Work out the finished part from the listing and answer in its coordinate system (mm). A direction names the side the tool comes from. Coordinates: 2 decimals unless noted, no trailing zeros. Order: outer loops, then holes, each group sorted by start corner. A loop starts at its lowest first (then second) coordinate and runs counter-clockwise, first axis right, second up. Notation, with made-up numbers: M -24.5,46.5 L 10.5,46.5 A29 ccw 10.5,85.5 Z; hole C 26.5,-7 d2. An arc over 180 degrees is marked long. Use a Markdown table: item, result.
from build123d import *

# Parameters (mm, degrees)
Y_KSEKLIK_EKSTR_ZYON1_DEPTH = 38
RADYUS3_R                   = 8
Y_KSEKLIK_EKSTR_ZYON2_DEPTH = 10
Y_KSEKLIK_EKSTR_ZYON3_DEPTH = 24
KES_EKSTR_ZYON1_DEPTH       = 68
KES_EKSTR_ZYON3_DEPTH       = 68
KES_EKSTR_ZYON3_DEPTH_BACK  = 68
KES_EKSTR_ZYON4_DEPTH       = 68
KES_EKSTR_ZYON7_DEPTH       = 68


with BuildPart() as part:
    # Çizim1 → Yükseklik-Ekstrüzyon1 (new body)
    with BuildSketch(Plane.XY):
        with BuildLine():
            Line((-8, 0), (-24, 0))
            Line((-24, 0), (-24, -12))
            Line((-24, -12), (-19.5, -18))
            Line((-19.5, -18), (-12.5, -18))
            Line((-12.5, -18), (-10.25, -15))
            Line((-10.25, -15), (10.25, -15))
            Line((10.25, -15), (12.5, -18))
            Line((12.5, -18), (19.5, -18))
            Line((19.5, -18), (24, -12))
            Line((24, -12), (24, 0))
            Line((24, 0), (8, 0))
            ThreePointArc((8, 0), (0, -8), (-8, 0))
        make_face()
    extrude(amount=Y_KSEKLIK_EKSTR_ZYON1_DEPTH)

    # Radyus3
    # the kernel refuses this fillet: 8 mm, written as the material it adds along each edge
    with BuildSketch(Plane(origin=(10.25, -15, 0), x_dir=(-1, 0, 0), z_dir=(0, 0, 1))) as radyus3_piece_1:
        with BuildLine():
            CenterArc((3.994997998, 8), RADYUS3_R, 218.682187453, 51.317812547)
            Line((-2.25, 3), (-2.37489996, 2.9))
            ThreePointArc((-2.37489996, 2.9), (-1.253, 1.404), (-0.128, -0.096))
            Line((-0.128, -0.096), (0, -0.16))
            Line((0, -0.16), (3.994997998, -0.16))
            Line((3.994997998, -0.16), (3.994997998, 0))
        make_face()
    extrude(amount=38)
    with BuildSketch(Plane(origin=(-10.25, -15, 0), x_dir=(-0.5999999999999978, -0.8000000000000017, 0), z_dir=(0, 0, 1))) as radyus3_piece_2:
        with BuildLine():
            CenterArc((4.003001201, 7.995998399), RADYUS3_R, 216.869897646, 51.317812547)
            Line((-2.396998799, 3.195998399), (-2.524998799, 3.099998399))
            Line((-2.524998799, 3.099998399), (-0.128, -0.096))
            Line((-0.128, -0.096), (0, -0.16))
            ThreePointArc((0, -0.16), (1.875, -0.16), (3.744939976, -0.159919968))
            Line((3.744939976, -0.159919968), (3.75, 0))
        make_face()
    extrude(amount=38)

    # Çizim2 → Yükseklik-Ekstrüzyon2 (add)
    with BuildSketch(Plane.XY.offset(38)):
        with BuildLine():
            Line((22.125, -12), (24, -12))
            Line((24, -12), (24, 0))
            Line((24, 0), (-24, 0))
            Line((-24, 0), (-24, -12))
            Line((-24, -12), (-22.125, -12))
            Line((-22.125, -12), (-18.75, -16.5))
            Line((-18.75, -16.5), (-13.183205232, -16.5))
            ThreePointArc((-13.183205232, -16.5), (-10.029919219, -14.282202113), (-6.255002002, -13.5))
            Line((-6.255002002, -13.5), (6.255002002, -13.5))
            ThreePointArc((6.255002002, -13.5), (10.029919219, -14.282202113), (13.183205232, -16.5))
            Line((13.183205232, -16.5), (18.75, -16.5))
            Line((18.75, -16.5), (22.125, -12))
        make_face()
    extrude(amount=Y_KSEKLIK_EKSTR_ZYON2_DEPTH)

    # Çizim4 → Yükseklik-Ekstrüzyon3 (add, symmetric)
    with BuildSketch(Plane(origin=(0, 0, 0), x_dir=(0, 0, -1), z_dir=(1, 0, 0))):
        Polygon((-109, -10.5), (-103, -16.5), (-48, -16.5), (-48, 0), (-98, 0), (-98, 5.5), (-103, 5.5), (-109, -0.5), align=None)
    extrude(amount=Y_KSEKLIK_EKSTR_ZYON3_DEPTH, both=True)

    # Çizim5 → Kes-Ekstrüzyon1 (cut)
    with BuildSketch(Plane(origin=(0, 0, 48), x_dir=(-1, 0, 0), z_dir=(0, 0, -1))):
        Polygon((24, -16.5), (24, -12), (22.125, -12), (18.75, -16.5), align=None)
    extrude(amount=-KES_EKSTR_ZYON1_DEPTH, mode=Mode.SUBTRACT)

    # Çizim6 → Kes-Ekstrüzyon3 (cut, two sides: drawn at the far end of the back side and taken through both)
    with BuildSketch(Plane(origin=(0, 0, 0), x_dir=(1, 0, 0), z_dir=(0, 1, 0)).offset(-KES_EKSTR_ZYON3_DEPTH_BACK)):
        Polygon((-24, -83.22), (-34.13268128, -83.22), (-34.13268128, -122.200491655), (32.816911355, -122.200491655), (32.816911355, -83.22), (24, -83.22), (12, -104.004609691), (-12, -104.004609691), align=None)
    extrude(amount=KES_EKSTR_ZYON3_DEPTH + KES_EKSTR_ZYON3_DEPTH_BACK, mode=Mode.SUBTRACT)

    # Çizim7 → Kes-Ekstrüzyon4 (cut)
    with BuildSketch(Plane(origin=(0, 0, 48), x_dir=(-1, 0, 0), z_dir=(0, 0, -1))):
        with BuildLine():
            Line((6.255002002, -13.5), (-6.255002002, -13.5))
            ThreePointArc((-6.255002002, -13.5), (-10.029919219, -14.282202113), (-13.183205232, -16.5))
            Line((-13.183205232, -16.5), (13.183205232, -16.5))
            ThreePointArc((13.183205232, -16.5), (10.029919219, -14.282202113), (6.255002002, -13.5))
        make_face()
        Polygon((-24, -16.5), (-18.75, -16.5), (-22.125, -12), (-24, -12), align=None)
    extrude(amount=-KES_EKSTR_ZYON4_DEPTH, mode=Mode.SUBTRACT)

    # Çizim9 → Kes-Ekstrüzyon7 (cut)
    with BuildSketch(Plane(origin=(0, 0, 0), x_dir=(1, 0, 0), z_dir=(0, 1, 0))):
        Polygon((0, -47.215390309), (-18, -57.607695155), (-18, -78.392304845), (0, -88.784609691), (18, -78.392304845), (18, -57.607695155), align=None)
    extrude(amount=-KES_EKSTR_ZYON7_DEPTH, mode=Mode.SUBTRACT)


solid = part.part
(1) A cutting plane is placed at B-B (y = -10.75). Determine the outline of the cut face in (x, z).
Conclusion:
| item | result |
|---|---|
| outline | M -24,0 L 24,0 L 24,83.22 L 12,104 L -12,104 L -24,83.22 Z; hole M -18,57.61 L 0,47.22 L 18,57.61 L 18,78.39 L 0,88.78 L -18,78.39 Z |
(2) A cutting plane is placed at D-D (y = 3.5). Determine the outline of the cut face in (x, z), then the cut area to 3 significant figures.
Conclusion:
| item | result |
|---|---|
| outline | M -15.47,98 L 15.47,98 L 12,104 L -12,104 Z |
| area | 165 mm2 |
(3) Straight lines are drawn through the part: L1, parallel to X at y = -8.25, z = 62; L2, parallel to Z at x = 0, y = -1.25; L3, parallel to Z at x = 0, y = -9. For each, find the intervals that lie inside material, in ascending order.
Conclusion:
| item | result |
|---|---|
| L1 | -24 to -18, 18 to 24 |
| L2 | 38 to 47.22, 88.78 to 104 |
| L3 | 0 to 47.22, 88.78 to 104 |
(4) Which of the six approach directions +Z, -Z, +X, -X, +Y, -Y give full straight-line access (tool end or side, diameter ignored) to faces 4 (the flat face through (0, -13.5, 94)), 5 (the cylindrical face through (0, -8, 19)), 6 (the flat face through (23, -12, 62)), 7 (the flat face through (0, 3, 98)), 8 (the flat face through (-9.126, -6.301, 83.516))?
Conclusion:
| item | result |
|---|---|
| face 4 | +Z, -Y |
| face 5 | -Z, +Y |
| face 6 | +Z, +X, -Y |
| face 7 | -Z, +X, -X, +Y |
| face 8 | +Y, -Y |
(5) A cutting plane is placed at C-C (z = 15). Determine the outline of the cut face in (x, y) (3 decimals).
Conclusion:
| item | result |
|---|---|
| outline | M -24,-12 L -19.5,-18 L -12.5,-18 A8 cw -6.255,-15 L 6.255,-15 A8 cw 12.5,-18 L 19.5,-18 L 24,-12 L 24,0 L 8,0 A8 cw -8,0 L -24,0 Z |
(6) A cutting plane is placed at A-A (z = 63.5). Determine the outline of the cut face in (x, y) (3 decimals), then the cut area to 3 significant figures.
Conclusion:
| item | result |
|---|---|
| outline | M -24,-12 L -22.125,-12 L -18.75,-16.5 L -18,-16.5 L -18,0 L -24,0 Z; M 18,-16.5 L 18.75,-16.5 L 22.125,-12 L 24,-12 L 24,0 L 18,0 Z |
| area | 166 mm2 |
(7) Determine the mould class of faces 1 (the flat face through (18.5, -16.5, 70.4)), 2 (the flat face through (9.126, -6.301, 52.484)), 3 (the flat face through (24, -6, 42)) for opening direction X: pulls with the +X half, pulls with the -X half, needs draft (parallel to the pull), parting line crosses it, or undercut.
Conclusion:
| item | result |
|---|---|
| face 1 | needs draft |
| face 2 | undercut |
| face 3 | pulls with the +X half |
(8) Given P1, Ø0.6, axis at x = 23, z = 72.5, coming from the -Y side; P2, Ø4, axis at x = 2, z = 94, coming from the -Y side; P3, Ø6, axis at x = -16, z = 74, coming from the -Y side; P4, Ø14.5, axis at x = -3.5, z = 71.5, coming from the +Y side (1 decimal), each flat-ended and moving along its own axis, determine where each tip first touches the part or whether it passes through.
Conclusion:
| item | result |
|---|---|
| P1 | y = -12 |
| P2 | y = -13.5 |
| P3 | y = -16.5 |
| P4 | through |
